from build123d import *

# Parameters (mm, degrees)
SKETCH1_W               = 76.2
SKETCH1_H               = 50.8
BOSS_EXTRUDE1_DEPTH     = 12.7
SKETCH2_R               = 3.175
CUT_EXTRUDE1_DEPTH      = 65.757547823
SKETCH3_R               = 4.7625
CUT_EXTRUDE2_DEPTH      = 65.757547823
F_1_4_CLEARANCE_HOLE1_D = 6.7564
F_8_CLEARANCE_HOLE1_D   = 4.4958
SKETCH10_R              = 3.81
CUT_EXTRUDE3_DEPTH      = 4.572
SKETCH11_R              = 6.096
CUT_EXTRUDE4_DEPTH      = 3.556


with BuildPart() as part:
    # Sketch1 → Boss-Extrude1 (new body)
    with BuildSketch(Plane(origin=(0, 0, 0), x_dir=(1, 0, 0), z_dir=(0, 1, 0))):
        Rectangle(SKETCH1_W, SKETCH1_H)
    extrude(amount=BOSS_EXTRUDE1_DEPTH)

    # Sketch2 → Cut-Extrude1 (cut, through all)
    with BuildSketch(Plane.XY.offset(25.4)):
        with Locations((-25.4, 0)):
            Circle(SKETCH2_R)
        with Locations((25.4, 0)):
            Circle(SKETCH2_R)
    extrude(amount=-CUT_EXTRUDE1_DEPTH, mode=Mode.SUBTRACT)

    # Sketch3 → Cut-Extrude2 (cut, through all)
    with BuildSketch(Plane.XY.offset(25.4)):
        with Locations((-9.525, 0)):
            Circle(SKETCH3_R)
        with Locations((9.525, 0)):
            Circle(SKETCH3_R)
    extrude(amount=-CUT_EXTRUDE2_DEPTH, mode=Mode.SUBTRACT)

    # 1/4 Clearance Hole1 (through all)
    with Locations(Plane(origin=(0, 12.7, 0), x_dir=(1, 0, 0), z_dir=(0, 1, 0))):
        with Locations((-33.3375, -19.05), (-33.3375, 19.05), (33.3375, 19.05), (33.3375, -19.05)):
            Hole(F_1_4_CLEARANCE_HOLE1_D / 2)

    # #8 Clearance Hole1 (through all)
    with Locations(Plane(origin=(0, 12.7, 0), x_dir=(1, 0, 0), z_dir=(0, 1, 0))):
        with Locations((-19.05, 19.05), (-19.05, -19.05), (19.05, -19.05), (19.05, 19.05), (0, 12.7), (0, -12.7)):
            Hole(F_8_CLEARANCE_HOLE1_D / 2)

    # Sketch10 → Cut-Extrude3 (cut)
    with BuildSketch(Plane(origin=(0, 12.7, 0), x_dir=(1, 0, 0), z_dir=(0, 1, 0))):
        with Locations(Location((0, 12.7, 0), (0, 0, 270))):
            Circle(SKETCH10_R)
        with Locations(Location((0, -12.7, 0), (0, 0, 270))):
            Circle(SKETCH10_R)
    extrude(amount=-CUT_EXTRUDE3_DEPTH, mode=Mode.SUBTRACT)

    # Sketch11 → Cut-Extrude4 (cut)
    with BuildSketch(Plane(origin=(0, 12.7, 0), x_dir=(1, 0, 0), z_dir=(0, 1, 0))):
        with Locations(Location((-19.05, 19.05, 0), (0, 0, 270))):
            Circle(SKETCH11_R)
        with Locations(Location((-19.05, -19.05, 0), (0, 0, 270))):
            Circle(SKETCH11_R)
        with Locations(Location((19.05, -19.05, 0), (0, 0, 270))):
            Circle(SKETCH11_R)
        with Locations(Location((19.05, 19.05, 0), (0, 0, 270))):
            Circle(SKETCH11_R)
    extrude(amount=-CUT_EXTRUDE4_DEPTH, mode=Mode.SUBTRACT)


solid = part.part
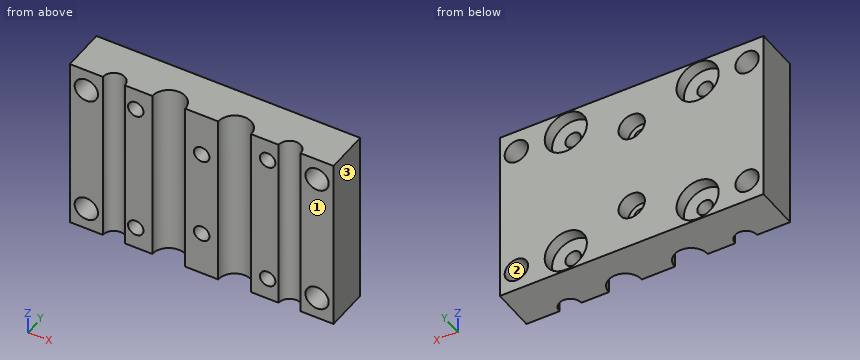
Geometry: final body of the model. Coordinates: model frame, mm. Face numbers are marked on the shaded views. Round coordinates to 2 decimals unless told otherwise and drop trailing zeros. Order: outer loops, then holes, each group sorted by start corner. A loop starts at its lowest first (then second) coordinate and runs counter-clockwise, first axis right, second up.
Q1. Section D-D, the plane x = 32. Output: boundary loops of the cut face in (y, z), and give its area (3 significant figures).
Result sheet:
outline: (0, -25.4) - (12.7, -25.4) - (12.7, -22.15) - (0, -22.15) - close; (0, -15.95) - (12.7, -15.95) - (12.7, 15.95) - (0, 15.95) - close; (0, 22.15) - (12.7, 22.15) - (12.7, 25.4) - (0, 25.4) - close
area: 488 mm2
Q2. Section B-B, the plane y = 11.5. Give the number of separate pieces and of enclosed holes in the cut face, and give its area (3 significant figures).
Result sheet:
separate pieces: 1
enclosed holes: 10
area: 3,170 mm2
Q3. Mould query, pull axis X, two halves, no side actions, for the marked faces 1, 2 and 3. Classes: released by +X, released by -X, zero draft, split by the parting line, or undercut.
Result sheet:
face 1: zero draft
face 2: undercut
face 3: released by +X
Q4. Pin query (flat end, axial travel): pin 1 (3.5 mm diameter, centred on x = 20, z = 16.5, fed in from +Y); pin 2 (6 mm diameter, centred on x = -0.5, z = -12.5, fed in from +Y); pin 3 (4 mm diameter, centred on x = 0, z = 12.7, fed in from -Y). Return the tip coordinate at first contact, or that it passes through.
Result sheet:
pin 1: stops at y = 9.14
pin 2: stops at y = 8.13
pin 3: passes through
Q5. Material intervals for probe 1 along X at (y, z) = (10.4, -19.05); probe 2 along X at (y, z) = (5, 19.05); probe 3 along Z at (x, y) = (14.5, 11.75), sorted ascending.
Result sheet:
probe 1: x = -38.1 to -36.72, -29.96 to -25.15, -12.95 to 12.95, 25.15 to 29.96, 36.72 to 38.1
probe 2: x = -38.1 to -36.72, -29.96 to -21.3, -16.8 to 16.8, 21.3 to 29.96, 36.72 to 38.1
probe 3: z = -25.4 to -23.11, -14.99 to 14.99, 23.11 to 25.4
Q6. Section A-A, the plane x = 19.05. Output: boundary loops of the cut face in (y, z).
Result sheet:
outline: (0, -25.4) - (12.7, -25.4) - (12.7, -25.15) - (9.14, -25.15) - (9.14, -21.3) - (0, -21.3) - close; (0, -16.8) - (9.14, -16.8) - (9.14, -12.95) - (12.7, -12.95) - (12.7, 12.95) - (9.14, 12.95) - (9.14, 16.8) - (0, 16.8) - close; (0, 21.3) - (9.14, 21.3) - (9.14, 25.15) - (12.7, 25.15) - (12.7, 25.4) - (0, 25.4) - close
